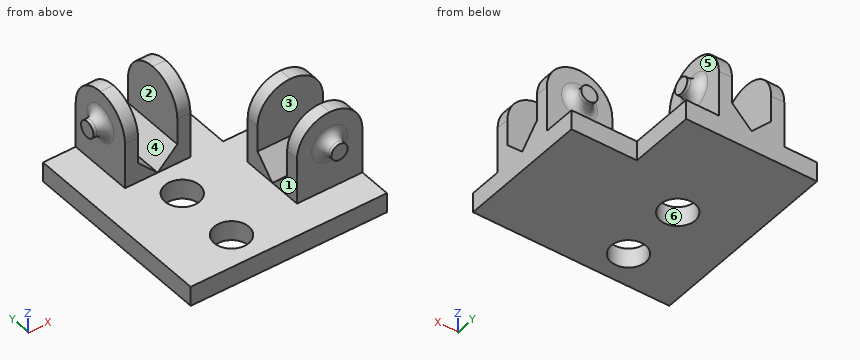
```python
from build123d import *

# Parameters (mm, degrees)
SKETCH1_W           = 20
SKETCH1_H           = 30
SKETCH1_R           = 2.65
SKETCH1_W_2         = 10
SKETCH1_H_2         = 20
BOSS_EXTRUDE1_DEPTH = 3
SKETCH2_W           = 10
SKETCH2_H           = 2
SKETCH2_W_2         = 2
SKETCH2_H_2         = 10
BOSS_EXTRUDE2_DEPTH = 12
FILLET1_R           = 5
SKETCH3_R           = 1.25
BOSS_EXTRUDE3_DEPTH = 2
BOSS_EXTRUDE4_START = -12
SKETCH3_2_R         = 1.25
BOSS_EXTRUDE4_DEPTH = 2
SKETCH4_R           = 1.25
BOSS_EXTRUDE5_DEPTH = 2
BOSS_EXTRUDE6_START = -12
SKETCH4_3_R         = 1.25
BOSS_EXTRUDE6_DEPTH = 2
FILLET2_R           = 1.5
CHAMFER1_SIZE       = 3


with BuildPart() as part:
    # Sketch1 → Boss-Extrude1 (new body)
    # profile 1 of 2: a face of its own
    with BuildSketch(Plane.XY):
        Rectangle(SKETCH1_W, SKETCH1_H)
        Circle(SKETCH1_R, mode=Mode.SUBTRACT)
        with Locations((0, -10)):
            Circle(SKETCH1_R, mode=Mode.SUBTRACT)
    # profile 2 of 2: a face of its own
    with BuildSketch(Plane.XY):
        with Locations((15, -5)):
            Rectangle(SKETCH1_W_2, SKETCH1_H_2)
    extrude(amount=BOSS_EXTRUDE1_DEPTH)

    # Sketch2 → Boss-Extrude2 (add)
    with BuildSketch(Plane.XY.offset(3)):
        with Locations((15, -9)):
            Rectangle(SKETCH2_W, SKETCH2_H)
        with Locations((15, -1)):
            Rectangle(SKETCH2_W, SKETCH2_H)
        with Locations((4, 10)):
            Rectangle(SKETCH2_W_2, SKETCH2_H_2)
        with Locations((-4, 10)):
            Rectangle(SKETCH2_W_2, SKETCH2_H_2)
    extrude(amount=BOSS_EXTRUDE2_DEPTH)

    # Fillet1
    fillet1_edges = [part.edges().sort_by_distance(p)[0] for p in [
        (-4, 15, 15),
        (-4, 5, 15),
        (4, 15, 15),
        (4, 5, 15),
        (10, -1, 15),
        (20, -1, 15),
        (20, -9, 15),
        (10, -9, 15),
    ]]
    fillet(fillet1_edges, radius=FILLET1_R - 0.0001)  # a hair under: the kernel refuses the full size

    # Sketch3 → Boss-Extrude3 (add)
    with BuildSketch(Plane.XZ.offset(10)):
        with Locations(Location((15, 10, 0), (0, 0, 180))):
            Circle(SKETCH3_R)
    extrude(amount=BOSS_EXTRUDE3_DEPTH)

    # Sketch3<2> → Boss-Extrude4 (add)
    with BuildSketch(Plane.XZ.offset(10).offset(BOSS_EXTRUDE4_START)):
        with Locations(Location((15, 10, 0), (0, 0, 180))):
            Circle(SKETCH3_2_R)
    extrude(amount=BOSS_EXTRUDE4_DEPTH)

    # Sketch4 → Boss-Extrude5 (add)
    with BuildSketch(Plane(origin=(5, 0, 0), x_dir=(0, 0, -1), z_dir=(1, 0, 0))):
        with Locations(Location((-10, 10, 0), (0, 0, 270))):
            Circle(SKETCH4_R)
    extrude(amount=BOSS_EXTRUDE5_DEPTH)

    # Sketch4<3> → Boss-Extrude6 (add)
    with BuildSketch(Plane(origin=(5, 0, 0), x_dir=(0, 0, -1), z_dir=(1, 0, 0)).offset(BOSS_EXTRUDE6_START)):
        with Locations(Location((-10, 10, 0), (0, 0, 270))):
            Circle(SKETCH4_3_R)
    extrude(amount=BOSS_EXTRUDE6_DEPTH)

    # Fillet2
    fillet2_edges = [part.edges().sort_by_distance(p)[0] for p in [
        (16.25, -10, 10),
        (16.25, 0, 10),
        (5, 11.25, 10),
        (-5, 11.25, 10),
    ]]
    fillet(fillet2_edges, radius=FILLET2_R)

    # Chamfer1
    chamfer1_edges = [part.edges().sort_by_distance(p)[0] for p in [
        (15, -8, 3),
        (15, -2, 3),
        (-3, 10, 3),
        (3, 10, 3),
    ]]
    chamfer(chamfer1_edges, length=CHAMFER1_SIZE - 0.0001)  # a hair under: the kernel refuses the full size


solid = part.part
```
Input: part model. Units: mm. Frame: model coordinates. Face numbers are marked on the shaded views. A direction names the side the tool comes from. Give positions to 0.01 mm unless a question says otherwise; leave off trailing zeros. Write each loop counter-clockwise with the first axis right and the second up, starting at its lowest first coordinate (ties: lowest second). Pieces come first, ordered by that corner, then holes. Notation, with made-up numbers: (43, -30) - (61, -30) arc R23 cw to (61, 7) - close; hole circle Ø5 at (52, 63.25). An arc over 180 degrees is marked (long way). Write item = value, one per line. Start each with the question number.
1) Cut plane C-C (z = 3.75). Return loops of the section in (x, y).
2) Reachability of the marked faces 1, 2 and 3 from +Z, -Z, +X, -X, +Y, -Y: full face, straight path, thin tool, end or side. Return the list, or none.
3) Material intervals for L1, parallel to Y at x = 0, z = 2.25; L2, parallel to Y at x = -1.25, z = 1.25; L3, parallel to X at y = 13.25, z = 11.25, sorted ascending. Write a range as [from, to].
4) Pin query (flat end, axial travel): pin 1 (4 mm diameter, centred on x = 1.5, z = 7, fed in from -Y); pin 2 (3 mm diameter, centred on y = 10, z = 8, fed in from -X); pin 3 (15 mm diameter, centred on x = -0.5, y = -5.5, fed in from +Z); pin 4 (2 mm diameter, centred on y = -6, z = 6.5, fed in from -X). Return the tip coordinate at first contact, or that it passes through.
5) Draft query along Z for the marked faces 4, 5 and 6. Return one class per face: pulls with the +Z half, pulls with the -Z half, needs draft (parallel to the pull), parting line crosses it, or undercut.
6) Cut plane A-A (z = 6.5). Return loops of the section in (x, y), and give its area (3 significant figures).
7) Cut plane B-B (x = 1.75). Return loops of the section in (y, z).
Answers follow:
q1.outline = (-5, 5) - (-0.75, 5) - (-0.75, 15) - (-5, 15) - close; (0.75, 5) - (5, 5) - (5, 15) - (0.75, 15) - close; (10, -10) - (20, -10) - (20, -5.75) - (10, -5.75) - close; (10, -4.25) - (20, -4.25) - (20, 0) - (10, 0) - close
q2.face_1 = +Z, -X, +Y, -Y
q2.face_2 = +Z, +Y, -Y
q2.face_3 = +Z, +X, -X
q3.L1 = [-15, -12.65], [-7.35, -2.65], [2.65, 15]
q3.L2 = [-15, -12.34], [-7.66, -2.34], [2.34, 15]
q3.L3 = [-5, -3], [3, 5]
q4.pin_1 = 5
q4.pin_2 = -7
q4.pin_3 = 3
q4.pin_4 = through
q5.face_4 = pulls with the +Z half
q5.face_5 = undercut
q5.face_6 = needs draft
q6.outline = (-5, 5) - (-3, 5) - (-3, 15) - (-5, 15) - close; (3, 5) - (5, 5) - (5, 15) - (3, 15) - close; (10, -10) - (20, -10) - (20, -8) - (10, -8) - close; (10, -2) - (20, -2) - (20, 0) - (10, 0) - close
q6.area = 80.0 mm^2
q7.outline = (-15, 0) - (-11.99, 0) - (-11.99, 3) - (-15, 3) - close; (-8.01, 0) - (-1.99, 0) - (-1.99, 3) - (-8.01, 3) - close; (1.99, 0) - (15, 0) - (15, 4.75) - (5, 4.75) - (5, 3) - (1.99, 3) - close
